Print and shaded views of the part. All mm, measured from the part's lowest x, y and z. Round coordinates to 2 decimals unless told otherwise and drop trailing zeros. Order: outer loops, then holes, each group sorted by start corner. A loop starts at its lowest first (then second) coordinate and runs counter-clockwise, first axis right, second up. Notation, with made-up numbers: (43.25, 27.25) -> (59.25, 27.25) arc R10 ccw to (59.25, 45.25) -> close; hole circle Ø3 at (-26, 21.25). An arc over 180 degrees is marked (long way). Answer as CSV lines item,"result".
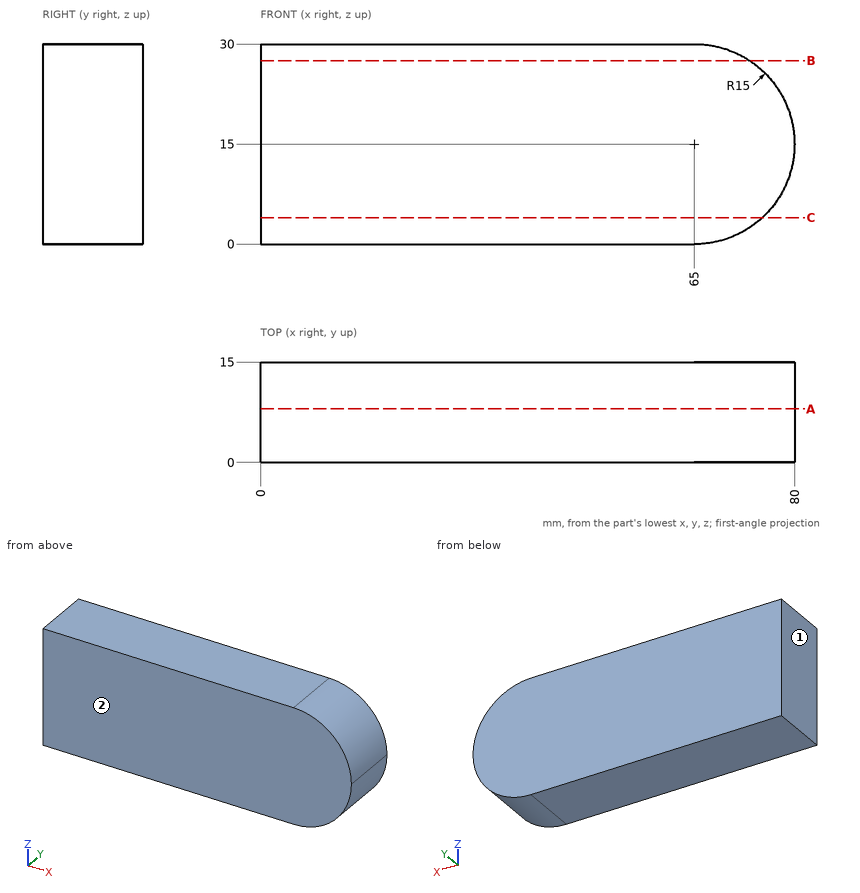
Q1. Saw through at A-A (y = 8). Write the cut outline in (x, z).
Checks:
outline,"(0, 0) -> (65, 0) arc R15 ccw to (65, 30) -> (0, 30) -> close"
Q2. Flat gauge pins, fed straight in: pin 1 (5 mm diameter, centred on x = 8.5, y = 2.5, fed in from -Z); pin 2 (1.5 mm diameter, centred on y = 12.5, z = 7, fed in from +X). Where does each tip first touch, or does it go through?
Checks:
pin 1,"z = 0"
pin 2,"x = 78.13"
Q3. Mould opens along X. For the marked faces 1 and 2 say: +X half, -X half, draft (parallel to the pull), parting line (faces both ways), or undercut.
Checks:
face 1,"-X half"
face 2,"draft"
Q4. Saw through at B-B (z = 27.5). Write the cut outline in (x, y), plus the area to 3 significant figures.
Checks:
outline,"(0, 0) -> (73.29, 0) -> (73.29, 15) -> (0, 15) -> close"
area,"1,100 mm²"
Q5. Wall check: L1, parallel to X at y = 9.5, z = 15.25; L2, parallel to X at y = 12.25, z = 2; L3, parallel to Z at x = 74, y = 1.25. Give the ranges that are in metal, low to high. Write a range as [from, to].
Checks:
L1,"[0, 80]"
L2,"[0, 72.48]"
L3,"[3, 27]"
Q6. Saw through at C-C (z = 4). Write the cut outline in (x, y).
Checks:
outline,"(0, 0) -> (75.2, 0) -> (75.2, 15) -> (0, 15) -> close"
